Study the drawing (mm; zero at the part's minimum x, y, z) and answer. A direction names the side the tool comes from. Coordinates: 2 decimals unless noted, no trailing zeros. Loops run counter-clockwise (first coordinate to the right, second up) from the corner with the lowest first, then second, coordinate; pieces in that order, holes last. Notation, with made-up numbers: (29.5, -22) - (78.5, -22) arc R7 cw to (78.5, -15) - close; hole circle Ø1 at (33.25, 45.5). An arc over 180 degrees is marked (long way). Use one line per item in the form item = value. Start each with the question number.
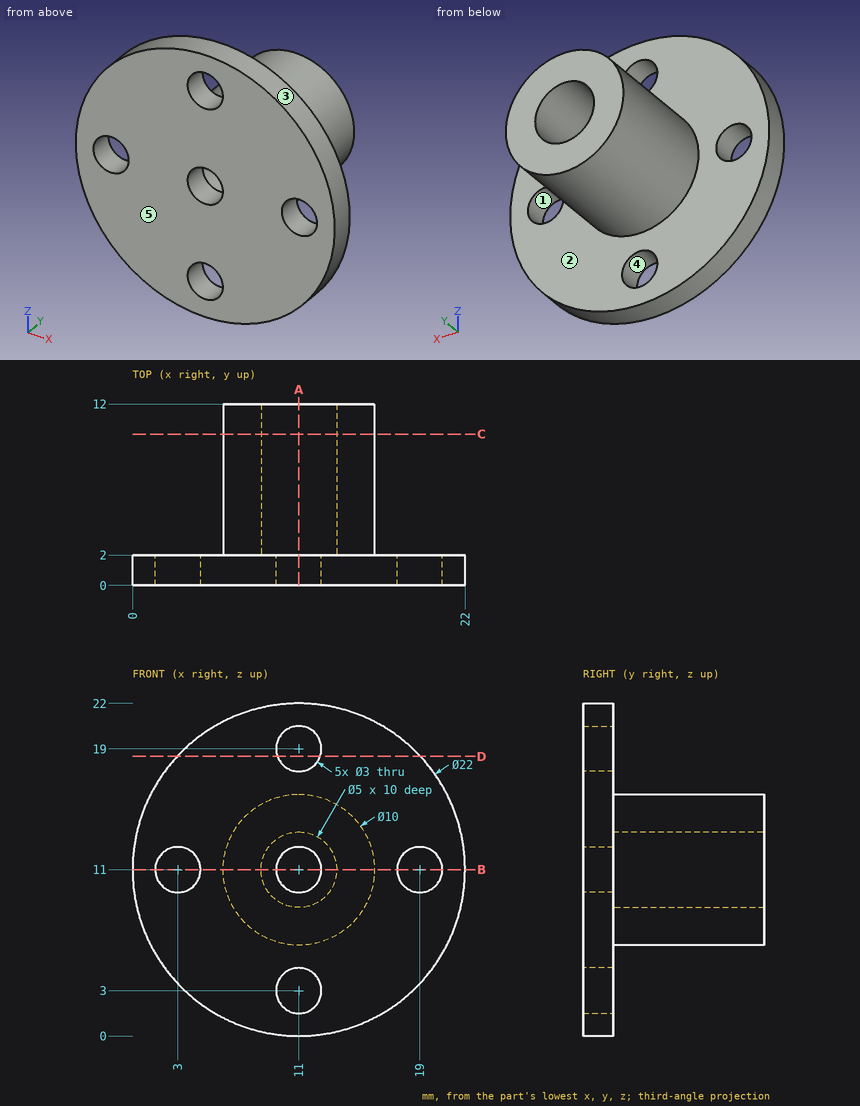
(1) A cutting plane is placed at D-D (z = 18.5). Determine the outline of the cut face in (x, y), then the cut area to 3 significant figures.
(2) For the marked faces 1 and 2, determine the directions among +Z, -Z, +X, -X, +Y, -Y from which every point of the face is accessible in a straight line to the end or side of a thin tool.
(3) Find the intervals of material crossed by probe 1 along X at (y, z) = (0.85, 11); probe 2 along X at (y, z) = (8.5, 11); probe 3 along Y at (x, z) = (7.5, 6.75), in increasing order. Write a range as from..to.
(4) Determine the mould class of the marked faces 3, 4 and 5 for opening direction Z: +Z half, -Z half, draft (parallel to the pull), parting line (faces both ways), or undercut.
(5) A cutting plane is placed at A-A (x = 11). Determine the outline of the cut face in (y, z), then the cut area to 3 significant figures.
(6) A cutting plane is placed at B-B (z = 11). Determine the outline of the cut face in (x, y).
(7) Each of these flat-tipped pins is pushed along its axis until it touches: pin 1 Ø6 at (x, z) = (19, 6.5) entering from +Y; pin 2 Ø1.5 at (y, z) = (7, 12) entering from -X. Where does it stop, or does it pass through?
(8) A cutting plane is placed at C-C (y = 10). Determine the outline of the cut face in (x, z).
Evaluation:
q1.outline = (2.95, 0) - (9.59, 0) - (9.59, 2) - (2.95, 2) - close; (12.41, 0) - (19.05, 0) - (19.05, 2) - (12.41, 2) - close
q1.area = 26.5 mm^2
q2.face_1 = +Y, -Y
q2.face_2 = +Y
q3.probe_1 = 0..1.5, 4.5..9.5, 12.5..17.5, 20.5..22
q3.probe_2 = 6..8.5, 13.5..16
q3.probe_3 = 0..2
q4.face_3 = parting line
q4.face_4 = undercut
q4.face_5 = draft
q5.outline = (0, 0) - (2, 0) - (2, 1.5) - (0, 1.5) - close; (0, 4.5) - (2, 4.5) - (2, 6) - (12, 6) - (12, 8.5) - (2, 8.5) - (2, 9.5) - (0, 9.5) - close; (0, 12.5) - (2, 12.5) - (2, 13.5) - (12, 13.5) - (12, 16) - (2, 16) - (2, 17.5) - (0, 17.5) - close; (0, 20.5) - (2, 20.5) - (2, 22) - (0, 22) - close
q5.area = 76.0 mm^2
q6.outline = (0, 0) - (1.5, 0) - (1.5, 2) - (0, 2) - close; (4.5, 0) - (9.5, 0) - (9.5, 2) - (8.5, 2) - (8.5, 12) - (6, 12) - (6, 2) - (4.5, 2) - close; (12.5, 0) - (17.5, 0) - (17.5, 2) - (16, 2) - (16, 12) - (13.5, 12) - (13.5, 2) - (12.5, 2) - close; (20.5, 0) - (22, 0) - (22, 2) - (20.5, 2) - close
q7.pin_1 = 2
q7.pin_2 = 6.01
q8.outline = circle Ø10 at (11, 11); hole circle Ø5 at (11, 11)
